Design review of the part shown in the three views and the two pictorial views. Dimensions are in mm from the part's minimum x, y and z. Coordinates: 2 decimals unless noted, no trailing zeros. Loops run counter-clockwise (first coordinate to the right, second up) from the corner with the lowest first, then second, coordinate; pieces in that order, holes last. Notation, with made-up numbers: (70.25, -22.5) - (77.25, -22.5) arc R16 cw to (77.25, -8.5) - close; hole circle Ø5 at (36, -10.5). An arc over 180 degrees is marked (long way). One line per item, written item: value. Start each with the question number.
1. Take a section at B-B, the plane z = 4.25. Count the separate pieces of the cut face and the enclosed holes in it, and give its area (3 significant figures).
2. Take a section at C-C, the plane y = 51.5. State the section outline as (x, z) points.
3. Insertion check: pin 1 (1.9 mm diameter, centred on y = 50, z = 3.5, fed in from +X). The pin has a flat end and moves straight along its axis. Give the tip position at first contact, or say it passes through.
4. To check wall thickness, follow line 1 (X direction, y = 20, z = 3.75); line 2 (Y direction, x = 85, z = 5.5). State the ranges of each line that lie inside material, in increasing order. Write a range as from..to.
5. Take a section at A-A, the plane y = 12.7. State the section outline as (x, z) points, and give its area (3 significant figures).
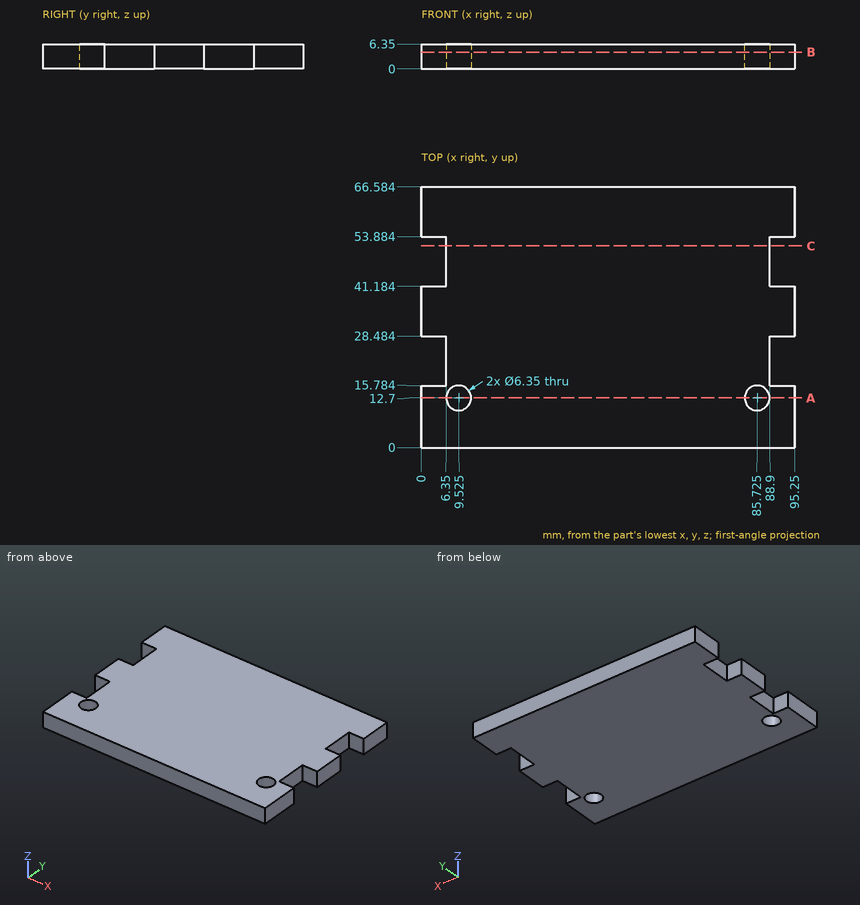
Solutions:
1. separate pieces: 1
1. enclosed holes: 2
1. area: 5,960 mm2
2. outline: (6.35, 0) - (88.9, 0) - (88.9, 6.35) - (6.35, 6.35) - close
3. pin 1: x = 88.9
4. line 1: 6.35..88.9
4. line 2: 0..9.61, 15.79..66.58
5. outline: (0, 0) - (6.35, 0) - (6.35, 6.35) - (0, 6.35) - close; (12.7, 0) - (82.55, 0) - (82.55, 6.35) - (12.7, 6.35) - close; (88.9, 0) - (95.25, 0) - (95.25, 6.35) - (88.9, 6.35) - close
5. area: 524 mm2
